Build history of the part. All positions in model axes, mm. A direction names the side the tool comes from. Give positions to 0.01 mm unless a question says otherwise; leave off trailing zeros. Loops run counter-clockwise (first coordinate to the right, second up) from the corner with the lowest first, then second, coordinate; pieces in that order, holes last.
1) Flat gauge pins, fed straight in: P1, Ø4.5, axis at x = 0, z = 0, coming from the +Y side; P2, Ø3.5, axis at x = 0, z = 0, coming from the +Y side; P3, Ø7.5, axis at x = -6, z = -6, coming from the -Y side. Where does each tip first touch, or does it go through?
2) Two-plate mould, pull along X, no slides. Class faces 4 (the cylindrical face through (-2.579, -23.888, 1.978)), 5 (the flat face through (0, -32, 0)), 6 (the cylindrical face through (0.07, -25.6, 1.5)): +X half, -X half, draft (parallel to the pull), parting line (faces both ways), or undercut.
3) Wall check: line 1 (Z direction, x = 0, y = -5); line 2 (Z direction, x = 0, y = -15.1); line 3 (Z direction, x = 0, y = -23.75). Give the ranges that are in metal, low to high.
4) Band-saw the part on B-B on y = -9. List the corners of the cut face in (x, z), then the cut area to 3 significant figures.
5) Band-saw the part on C-C on x = -9.5. List the corners of the cut face in (y, z).
6) 3-axis set-ups, long thin cutter, end or side, ignore diameter. For faces 1 (the cylindrical face through (10, -9.6, 3.2)), 2 (the cylindrical face through (2.764, 1.479, 12.447)), 3 (the flat face through (-2, -12.8, -1)): which of +Z, -Z, +X, -X, +Y, -Y reach the whole face in a straight line?
7) Band-saw the part on D-D on y = -27. List the corners of the cut face in (x, z), then the cut area to 3 significant figures.
Autodesk Inventor part; units mm, degrees
ref_plane "Arbeitsebene3" through (0, 0, 0) normal (1, 0, 0) x (0, 1, 0)
ref_plane "XZ Plane" through (0, 0, 0) normal (0, 1, 0) x (-1, 0, 0)
ref_plane "XY Plane" through (0, 0, 0) normal (0, 0, 1) x (1, 0, 0)
sketch "Skizze1" plane through (0, 0, 0) normal (0, 1, 0) x (-1, 0, 0)
  circle A0 centre (0, 0) radius 12.75
  dimension "d0" = 25.5
extrude "Extrusion1" add sketch "Skizze1" along normal blind 3
sketch "Skizze2" plane through (0, 0, 0) normal (0, -1, 0) x (1, 0, 0)
  circle A0 centre (0, 0) radius 12.25
  dimension "d3" = 24.5
extrude "Extrusion2" add sketch "Skizze2" along normal blind 16
sketch "Skizze6" plane through (0, -16, 0) normal (0, -1, 0) x (1, 0, 0)
  circle A0 centre (0, 0) radius 10.5
  dimension "d20" = 21
extrude "Extrusion5" cut sketch "Skizze6" against normal blind 13
sketch "Skizze7" plane through (0, -3, 0) normal (0, -1, 0) x (1, 0, 0)
  circle A0 centre (0, 0) radius 5.5
  dimension "d23" = 11
extrude "Extrusion6" add sketch "Skizze7" along normal up to surface (13 mm away)
sketch "Skizze8" plane through (0, -16, 0) normal (0, -1, 0) x (1, 0, 0)
  circle A0 centre (0, 0) radius 3.25
  dimension "d26" = 6.5
extrude "Extrusion7" add sketch "Skizze8" along normal blind 16
sketch "Skizze9" plane through (0, 3, 0) normal (0, 1, 0) x (1, 0, 0)
  circle A0 centre (0, 0) radius 12.75
hole "Bohrung2" at (0, 3, 0) direction (0, -1, 0) diameter 5 depth 15.8
ref_plane "Arbeitsebene3" through (0, 0, 0) normal (1, 0, 0) x (0, 1, 0)
sketch "Skizze11" plane through (0, 0, 0) normal (1, 0, 0) x (0, 1, 0)
  line L0 (-16, -3.25) -> (-32, -3.25)
  line L1 (-3, -5.5) -> (-16, -5.5)
  line L2 (-16, -5.5) -> (-16, 5.5)
  line L3 (-3, -10.5) -> (-3, 10.5)
  line L4 (-30.7422, 0) -> (0, 0)
  line L5 (-22.3, -2) -> (-12.8, -2)
  line L6 (-12.8, -2.5) -> (-12.8, 2.5)
  line L7 (-22.3, -2) -> (-22.3, -1.5)
  line L8 (-22.3, -1.5) -> (-28.8, -1.5)
  line L9 (-28.8, -1.5) -> (-28.8, 0)
  line L10 (-12.8, -2) -> (-12.8, 0)
  point P0 (-22.3, -1.75)
  point P1 (-16, -2)
  point P2 (-16, 0)
  dimension "d38" = 3
  dimension "d39" = 4
  dimension "d40" = 9.5
  dimension "d41" = 6.5
revolve "Umdrehung1" cut sketch "Skizze11" angle 360 about axis through (0, -30.7422, 0) along (0, 1, 0) contours L5 L7 L8 L9 L4 L2
sketch "Skizze14" plane through (0, -12.8, 0) normal (0, 1, 0) x (1, 0, 0)
  point P0 (0, 0)
  point P1 (0, 0)
hole "Bohrung4" at (0, -12.8, 0) direction (0, -1, 0) diameter 4 depth 5
properties part number "18" material "Gold"
Findings below:
1. P1: stops at y = -12.8
1. P2: stops at y = -22.3
1. P3: stops at y = -16
2. face 4: parting line
2. face 5: draft
2. face 6: undercut
3. line 1: z = -12.25 to -10.5, -5.5 to -2.5, 2.5 to 5.5, 10.5 to 12.25
3. line 2: z = -12.25 to -10.5, -5.5 to -2, 2 to 5.5, 10.5 to 12.25
3. line 3: z = -3.25 to -1.5, 1.5 to 3.25
4. outline: circle Ø24.5 at (0, 0); circle Ø11 at (0, 0); hole circle Ø21 at (0, 0); hole circle Ø5 at (0, 0)
4. area: 200 mm2
5. outline: (-16, -7.73) - (0, -7.73) - (0, -8.5) - (3, -8.5) - (3, 8.5) - (0, 8.5) - (0, 7.73) - (-16, 7.73) - (-16, 4.47) - (-3, 4.47) - (-3, -4.47) - (-16, -4.47) - close
6. face 1: -Y
6. face 2: +Y, -Y
6. face 3: +Y
7. outline: circle Ø6.5 at (0, 0); hole circle Ø3 at (0, 0)
7. area: 26.1 mm2
